from build123d import *

# Parameters (mm, degrees)
F2_R = 5
F3_R = 5


with BuildPart() as f1:
    # F0 (on Right) → F1 (revolve)
    with BuildSketch(Plane.YZ):
        Polygon((-39.0091740638, 9.247707203), (-26.0091740638, 9.247707203), (-13.0091740638, 9.247707203), (-13.0091740638, 10.247707203), (-15.0091740638, 10.247707203), (-15.0091740638, 11.247707203), (-22.9062791914, 11.247707203), (-24.0091740638, 16.747707203), (-25.0091740638, 16.747707203), (-26.0091740638, 15.4484901577), (-27.0091740638, 16.747707203), (-28.0091740638, 16.747707203), (-29.1120689362, 11.247707203), (-37.0091740638, 11.247707203), (-37.0091740638, 10.247707203), (-39.0091740638, 10.247707203), align=None)
    revolve(axis=Axis((0, -19.5091740638, 9.247707203), (0, 1, 0)))

    # F2
    f2_edges = [f1.edges().sort_by_distance(p)[0] for p in [
        (0, -29.112069, 7.247707),
    ]]
    fillet(f2_edges, radius=F2_R)

    # F3
    f3_edges = [f1.edges().sort_by_distance(p)[0] for p in [
        (0, -22.906279, 7.247707),
    ]]
    fillet(f3_edges, radius=F3_R)


solid = f1.part
Read the model definition and answer for the solid it produces. Units are mm, in the model's axes. A direction names the side the tool comes from. Give positions to 0.01 mm unless a question says otherwise; leave off trailing zeros. Loops run counter-clockwise (first coordinate to the right, second up) from the corner with the lowest first, then second, coordinate; pieces in that order, holes last. Notation, with made-up numbers: (69.25, 20.5) -> (75.25, 20.5) arc R14 cw to (75.25, 38.5) -> close; hole circle Ø5 at (5, 40.25). An arc over 180 degrees is marked (long way). Answer as CSV lines item,"result".
Item 1: Consider line 1 (Y direction, x = 5, z = 13.5); line 2 (X direction, y = -34, z = 8); line 3 (Y direction, x = 2, z = 11.75). Determine where each line is inside the solid, lowest interval first. Write a range as [from, to].
Returned:
line 1,"y = [-28.2, -26.29], [-25.73, -23.82]"
line 2,"x = [-1.56, 1.56]"
line 3,"y = [-29.96, -22.06]"
Item 2: Each of these flat-tipped pins is pushed along its axis until it touches: pin 1 (8 mm diameter, centred on x = 6, y = -28.5, fed in from -Z); pin 2 (1.5 mm diameter, centred on x = 2.5, y = -32.5, fed in from -Z); pin 3 (1.5 mm diameter, centred on x = 5.5, z = 9, fed in from -Y). Where does it stop, or does it pass through?
Returned:
pin 1,"stops at z = 2.03"
pin 2,"stops at z = 8.16"
pin 3,"stops at y = -28.74"
Item 3: For faces 1 (the face through (0.04, -14.02, 8.25)), 2 (the face through (0.04, -38.02, 8.25)), 3 (the face through (0, -39.009, 9)), determine the directions among +Z, -Z, +X, -X, +Y, -Y from which every point of the face is accessible in a straight line to the end or side of a thin tool.
Returned:
face 1,"+Y"
face 2,"-Y"
face 3,"+Z, -Z, +X, -X, -Y"
Item 4: Find section A-A on y = -35. Give the vertices of the cut face in (x, z), plus the area to 3 significant figures.
Returned:
outline,"circle Ø4 at (0, 9.25)"
area,"12.6 mm²"
